from build123d import *

# Parameters (mm, degrees)
SKETCH_1_R          = 5.5
EXTRUDE_1_DEPTH     = 5
EXTRUDE_START       = -5
EXTRUDE_2_DEPTH     = 5
CUT_EXTRUDE_1_REACH = 14.9


with BuildPart() as part:
    # 草图1 → 凸台-拉伸1 (new body)
    with BuildSketch(Plane(origin=(0, 0, 0), x_dir=(1, 0, 0), z_dir=(0, 1, 0))):
        with Locations(Location((0, 0, 0), (0, 0, 270))):
            Circle(SKETCH_1_R)
    extrude(amount=EXTRUDE_1_DEPTH)

    # 草图2 → 凸台-拉伸2 (add)
    with BuildSketch(Plane(origin=(0, 5, 0), x_dir=(-1, 0, 0), z_dir=(0, 1, 0)).offset(EXTRUDE_START)):
        with BuildLine():
            Line((-4.389411899, -7.317483391), (-5.60293739, -6.435805513))
            ThreePointArc((-5.60293739, -6.435805513), (-5.11774735, -4.915167527), (-3.987951794, -3.787643132))
            ThreePointArc((-3.987951794, -3.787643132), (-3.232818888, -4.449593469), (-2.369917805, -4.963213636))
            ThreePointArc((-2.369917805, -4.963213636), (-3.093131201, -6.386137262), (-4.389411899, -7.317483391))
        make_face()
        with BuildLine():
            Line((-7.852217643, -3.339936839), (-8.315743134, -1.913352065))
            ThreePointArc((-8.315743134, -1.913352065), (-7.029407564, -0.968317642), (-5.452641547, -0.720208411))
            ThreePointArc((-5.452641547, -0.720208411), (-5.23081084, -1.699593469), (-4.834607559, -2.622321444))
            ThreePointArc((-4.834607559, -2.622321444), (-6.256073009, -3.34839667), (-7.852217643, -3.339936839))
        make_face()
        with BuildLine():
            Line((-8.315743134, 1.913352065), (-7.852217643, 3.339936839))
            ThreePointArc((-7.852217643, 3.339936839), (-6.256073009, 3.34839667), (-4.834607559, 2.622321444))
            ThreePointArc((-4.834607559, 2.622321444), (-5.23081084, 1.699593469), (-5.452641547, 0.720208411))
            ThreePointArc((-5.452641547, 0.720208411), (-7.029407564, 0.968317642), (-8.315743134, 1.913352065))
        make_face()
        with BuildLine():
            Line((-5.60293739, 6.435805513), (-4.389411899, 7.317483391))
            ThreePointArc((-4.389411899, 7.317483391), (-3.093131201, 6.386137262), (-2.369917805, 4.963213636))
            ThreePointArc((-2.369917805, 4.963213636), (-3.232818888, 4.449593469), (-3.987951794, 3.787643132))
            ThreePointArc((-3.987951794, 3.787643132), (-5.11774735, 4.915167527), (-5.60293739, 6.435805513))
        make_face()
        with BuildLine():
            Line((-0.75, 8.5), (0.75, 8.5))
            ThreePointArc((0.75, 8.5), (1.251281594, 6.984590476), (1, 5.408326913))
            ThreePointArc((1, 5.408326913), (0, 5.5), (-1, 5.408326913))
            ThreePointArc((-1, 5.408326913), (-1.251281594, 6.984590476), (-0.75, 8.5))
        make_face()
        with BuildLine():
            Line((4.389411899, 7.317483391), (5.60293739, 6.435805513))
            ThreePointArc((5.60293739, 6.435805513), (5.11774735, 4.915167527), (3.987951794, 3.787643132))
            ThreePointArc((3.987951794, 3.787643132), (3.232818888, 4.449593469), (2.369917805, 4.963213636))
            ThreePointArc((2.369917805, 4.963213636), (3.093131201, 6.386137262), (4.389411899, 7.317483391))
        make_face()
        with BuildLine():
            Line((0.75, -8.5), (-0.75, -8.5))
            ThreePointArc((-0.75, -8.5), (-1.251281594, -6.984590476), (-1, -5.408326913))
            ThreePointArc((-1, -5.408326913), (0, -5.5), (1, -5.408326913))
            ThreePointArc((1, -5.408326913), (1.251281594, -6.984590476), (0.75, -8.5))
        make_face()
        with BuildLine():
            Line((7.852217643, 3.339936839), (8.315743134, 1.913352065))
            ThreePointArc((8.315743134, 1.913352065), (7.029407564, 0.968317642), (5.452641547, 0.720208411))
            ThreePointArc((5.452641547, 0.720208411), (5.23081084, 1.699593469), (4.834607559, 2.622321444))
            ThreePointArc((4.834607559, 2.622321444), (6.256073009, 3.34839667), (7.852217643, 3.339936839))
        make_face()
        with BuildLine():
            Line((8.315743134, -1.913352065), (7.852217643, -3.339936839))
            ThreePointArc((7.852217643, -3.339936839), (6.256073009, -3.34839667), (4.834607559, -2.622321444))
            ThreePointArc((4.834607559, -2.622321444), (5.23081084, -1.699593469), (5.452641547, -0.720208411))
            ThreePointArc((5.452641547, -0.720208411), (7.029407564, -0.968317642), (8.315743134, -1.913352065))
        make_face()
        with BuildLine():
            Line((5.60293739, -6.435805513), (4.389411899, -7.317483391))
            ThreePointArc((4.389411899, -7.317483391), (3.093131201, -6.386137262), (2.369917805, -4.963213636))
            ThreePointArc((2.369917805, -4.963213636), (3.232818888, -4.449593469), (3.987951794, -3.787643132))
            ThreePointArc((3.987951794, -3.787643132), (5.11774735, -4.915167527), (5.60293739, -6.435805513))
        make_face()
    extrude(amount=EXTRUDE_2_DEPTH)

    # 草图3 → 切除-拉伸1 (cut, up to next)
    with BuildSketch(Plane(origin=(0, 5, 0), x_dir=(-1, 0, 0), z_dir=(0, 1, 0)), mode=Mode.PRIVATE) as cut_extrude_1_sk1:
        with BuildLine():
            Line((1.25, -1.5612495), (1.25, 1.5612495))
            ThreePointArc((1.25, 1.5612495), (0, 2), (-1.25, 1.5612495))
            Line((-1.25, 1.5612495), (-1.25, -1.5612495))
            ThreePointArc((-1.25, -1.5612495), (0, -2), (1.25, -1.5612495))
        make_face()
    cut_extrude_1_tool1 = extrude(cut_extrude_1_sk1.sketch, amount=-CUT_EXTRUDE_1_REACH, mode=Mode.PRIVATE) & part.part
    add(cut_extrude_1_tool1.solids().sort_by_distance((0, 5, 0))[0], mode=Mode.SUBTRACT)


solid = part.part
Model file for the job. Use its own axes, mm. Round coordinates to 2 decimals unless told otherwise and drop trailing zeros. Loops run counter-clockwise (first coordinate to the right, second up) from the corner with the lowest first, then second, coordinate; pieces in that order, holes last. Notation, with made-up numbers: (57.5, 47.5) - (115.5, 47.5) arc R20 ccw to (115.5, 73.5) - close; hole circle Ø4 at (30, 58). An arc over 180 degrees is marked (long way). Write each question's results on one line, items separated by ' | '.
(1) Mould opens along X. For faces 1 (the cylindrical face through (-3.08, 2.46, 6.37)), 2 (the flat face through (-4.99, 2.46, 6.88)), 3 (the flat face through (0, 2, 8.5)), 4 (the cylindrical face through (-1.25, 2.46, 7.01)) say: released by +X, released by -X, zero draft, split by the parting line, or undercut.
Answer below:
face 1: undercut | face 2: released by -X | face 3: zero draft | face 4: undercut
(2) Saw through at C-C, the plane z = 4. List the corners of the cut face in (x, y).
Answer below:
outline: (-4.3, 0) - (4.3, 0) - (4.3, 5) - (-4.3, 5) - close
(3) Pin check, flat tip, straight feed: pin 1 (3 mm diameter, centred on y = 4, z = -5, fed in from -X). Stop position of the tip, or through.
Answer below:
pin 1: stops at x = -5.6
(4) Saw through at A-A, the plane z = 1. List the corners of the cut face in (x, y).
Answer below:
outline: (-7.1, 0) - (-1.25, 0) - (-1.25, 5) - (-7.1, 5) - close; (1.25, 0) - (7.1, 0) - (7.1, 5) - (1.25, 5) - close
(5) Wall check: L1, parallel to X at y = 4.7, z = -7.25; L2, parallel to Z at x = 5.25, y = 3.25; L3, parallel to Z at x = -5, y = 1.6. Give the ranges that are in metal, low to high.
Answer below:
L1: x = -4.48 to -4.23, -1.22 to 1.22, 4.23 to 4.48 | L2: z = -6.69 to -5.15, -2.93 to 2.93, 5.15 to 6.69 | L3: z = -6.87 to -4.74, -2.76 to 2.76, 4.74 to 6.87
(6) Saw through at B-B, the plane x = -1.75. List the corners of the cut face in (y, z), then the cut area to 3 significant figures.
Answer below:
outline: (0, -5.21) - (5, -5.21) - (5, 5.21) - (0, 5.21) - close | area: 52.1 mm^2
